Print and shaded views of the part. All mm, measured from the part's lowest x, y and z. A direction names the side the tool comes from. Round coordinates to 2 decimals unless told otherwise and drop trailing zeros. Loops run counter-clockwise (first coordinate to the right, second up) from the corner with the lowest first, then second, coordinate; pieces in that order, holes last. Notation, with made-up numbers: (37.25, 36) -> (46.25, 36) arc R21 cw to (46.25, 55) -> close; hole circle Ø11 at (31, 25). An arc over 180 degrees is marked (long way). Answer as CSV lines item,"result".
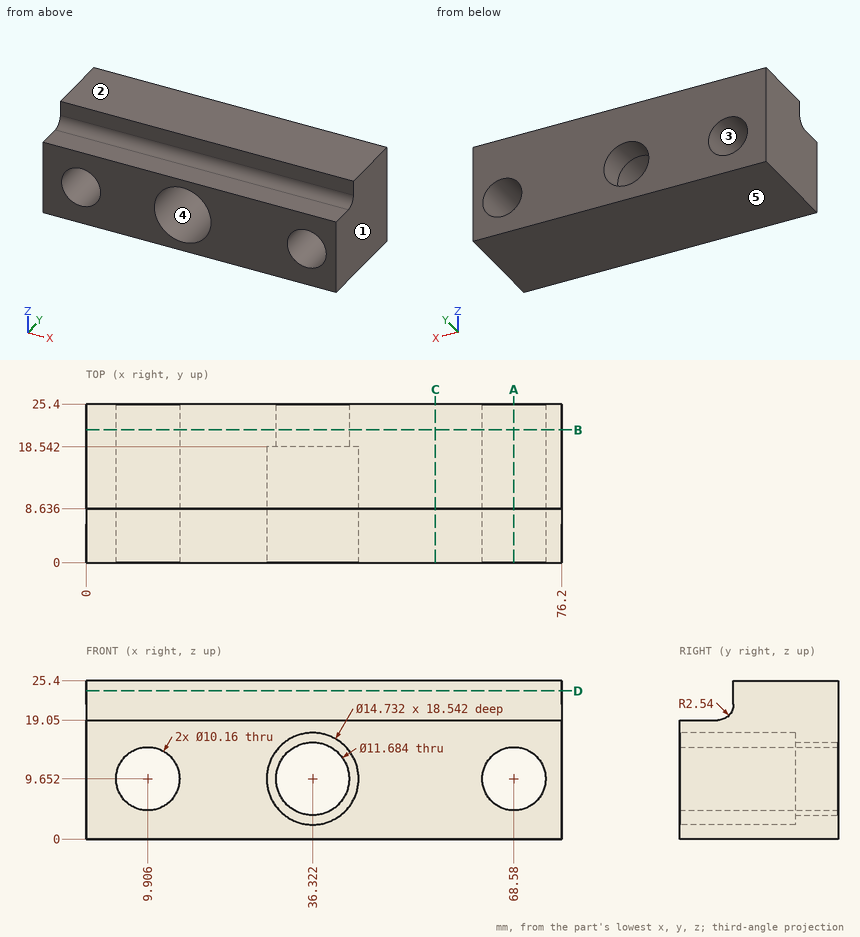
Q1. Slice it at D-D, the plane z = 23.75. Give the cut face in (x, y), and give its area (3 significant figures).
Results:
outline,"(0, 8.64) -> (76.2, 8.64) -> (76.2, 25.4) -> (0, 25.4) -> close"
area,"1,280 mm2"
Q2. Tool access for the marked faces 4 and 5: list every direction of +Z, -Z, +X, -X, +Y, -Y with a clear straight run to the whole face (end or side of a thin tool).
Results:
face 4,"-Y"
face 5,"-Z, +X, -X, +Y, -Y"
Q3. Drop flat-ended pins along their axis: pin 1 Ø3 at (x, z) = (35.5, 23) entering from -Y; pin 2 Ø9.5 at (x, z) = (36.322, 9.652) entering from -Y; pin 3 Ø1.8 at (x, y) = (33, 4) entering from +Z. Give the stop position or say it passes through.
Results:
pin 1,"y = 8.63"
pin 2,"through"
pin 3,"z = 19.05"
Q4. Two-plate mould, pull along X, no slides. Class the marked faces 1, 2 and 3: pulls with the +X half, pulls with the -X half, needs draft (parallel to the pull), parting line crosses it, or undercut.
Results:
face 1,"pulls with the +X half"
face 2,"needs draft"
face 3,"undercut"
Q5. Slice it at C-C, the plane x = 56. Give the cut face in (y, z), and give its area (3 significant figures).
Results:
outline,"(0, 0) -> (25.4, 0) -> (25.4, 25.4) -> (8.64, 25.4) -> (8.64, 21.59) arc R2.54 cw to (6.1, 19.05) -> (0, 19.05) -> close"
area,"592 mm2"
Q6. Slice it at A-A, the plane x = 68.58. Give the cut face in (y, z).
Results:
outline,"(0, 0) -> (25.4, 0) -> (25.4, 4.57) -> (0, 4.57) -> close; (0, 14.73) -> (25.4, 14.73) -> (25.4, 25.4) -> (8.64, 25.4) -> (8.64, 21.59) arc R2.54 cw to (6.1, 19.05) -> (0, 19.05) -> close"
Q7. Slice it at B-B, the plane y = 21.25. Give the cut face in (x, z), and give its area (3 significant figures).
Results:
outline,"(0, 0) -> (76.2, 0) -> (76.2, 25.4) -> (0, 25.4) -> close; hole circle Ø10.16 at (9.91, 9.65); hole circle Ø11.68 at (36.32, 9.65); hole circle Ø10.16 at (68.58, 9.65)"
area,"1,670 mm2"
Q8. Probe L1, parallel to X at y = 8.25, z = 5; L2, parallel to X at y = 11.5, z = 6; L3, parallel to Z at x = 68.58, y = 5.5. List the from-to ranges inside material, lowest first. Write a range as [from, to].
Results:
L1,"[0, 7.87], [11.95, 30.61], [42.03, 66.54], [70.62, 76.2]"
L2,"[0, 6.37], [13.44, 29.93], [42.72, 65.05], [72.11, 76.2]"
L3,"[0, 4.57], [14.73, 19.05]"
